Here's how the part is built. I have some questions about the finished solid (model axes, mm). Face numbers are marked on the shaded views. A direction names the side the tool comes from. Coordinates: 2 decimals unless noted, no trailing zeros. Write each loop counter-clockwise with the first axis right and the second up, starting at its lowest first coordinate (ties: lowest second). Pieces come first, ordered by that corner, then holes.
Item 1: For the marked faces 1 and 2, which set-ups out of +Z, -Z, +X, -X, +Y, -Y let a thin tool reach every point of the face, with its end or its side?
Item 2: If we section it at C-C (z = 23): Please give me the cut outline in (x, y).
Item 3: We'd pull the mould along Z, two halves only. Please class the marked faces 3, 4 and 5: +Z half, -Z half, draft (parallel to the pull), parting line (faces both ways), or undercut.
Item 4: If I drill on line 1 (Y direction, x = 12, z = -9); line 2 (Y direction, x = 22, z = 29); line 3 (Z direction, x = 0, y = -91.5), over which ranges is the centre line in solid material (lowest first)?
Item 5: If we section it at B-B (x = 0): Please give me the cut outline in (y, z), then the cut area to 3 significant figures.
Item 6: If we section it at D-D (y = -57.5): Please give me the cut outline in (x, z), then the cut area to 3 significant figures.
Item 7: I'm going to push flat-ended pins straight in: pin 1 Ø5 at (y, z) = (-63, -19.5) entering from -X; pin 2 Ø1.5 at (x, z) = (-12.5, 3.5) entering from -Y; pin 3 Ø10 at (x, z) = (35.96, -27.34) entering from +Y; pin 4 Ø6 at (x, y) = (24.5, -93.5) entering from -Z. Where does each tip first touch, or does it pass through?
Item 8: If we section it at A-A (z = 0): Please give me the cut outline in (x, y), then the cut area to 3 significant figures.
from build123d import *

# Parameters (mm, degrees)
F0_W     = 92.247778
F0_H     = 75.00481
F0_R     = 6.35
F1_DEPTH = 25.4
F2_R     = 31.75
F3_DEPTH = 76.2
F4_R     = 3.81
F5_DEPTH = 25.4


with BuildPart() as f1:
    # F0 (on Front) → F1 (new body)
    with BuildSketch(Plane.XZ):
        Rectangle(F0_W, F0_H)
        with Locations((-35.963889, -27.342405)):
            Circle(F0_R, mode=Mode.SUBTRACT)
        with Locations((35.963889, -27.342405)):
            Circle(F0_R, mode=Mode.SUBTRACT)
        with Locations((-35.963889, 27.342405)):
            Circle(F0_R, mode=Mode.SUBTRACT)
        with Locations((35.963889, 27.342405)):
            Circle(F0_R, mode=Mode.SUBTRACT)
    extrude(amount=F1_DEPTH)

    # F2 (on face) → F3 (join)
    with BuildSketch(Plane.XZ.offset(25.4)):
        Circle(F2_R)
    extrude(amount=F3_DEPTH)

    # F4 (on face) → F5 (join)
    with BuildSketch(Plane.XZ.offset(101.6)):
        Circle(F4_R)
    extrude(amount=F5_DEPTH)


solid = f1.part
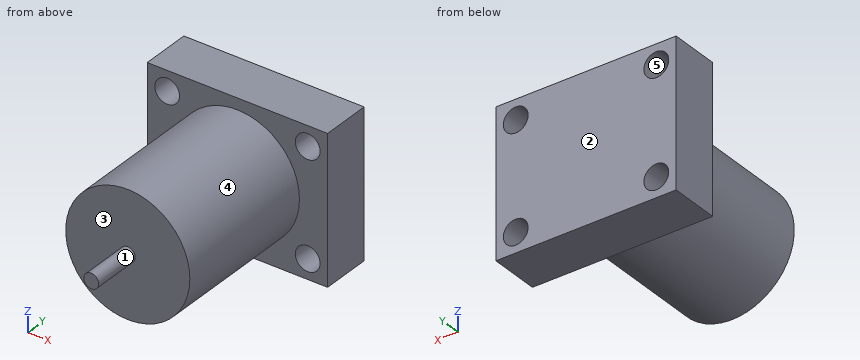
Answer list:
1. face 1: -Y
1. face 2: +Z, -Z, +X, -X, +Y
2. outline: (-46.12, -25.4) - (-40.6, -25.4) - (-40.6, 0) - (-46.12, 0) - close; (-31.33, -25.4) - (-21.89, -25.4) - (-21.89, -101.6) - (21.89, -101.6) - (21.89, -25.4) - (31.33, -25.4) - (31.33, 0) - (-31.33, 0) - close; (40.6, -25.4) - (46.12, -25.4) - (46.12, 0) - (40.6, 0) - close
3. face 3: draft
3. face 4: parting line
3. face 5: undercut
4. line 1: y = -101.6 to 0
4. line 2: y = -25.4 to 0
4. line 3: z = -31.75 to 31.75
5. outline: (-127, -3.81) - (-101.6, -3.81) - (-101.6, -31.75) - (-25.4, -31.75) - (-25.4, -37.5) - (0, -37.5) - (0, 37.5) - (-25.4, 37.5) - (-25.4, 31.75) - (-101.6, 31.75) - (-101.6, 3.81) - (-127, 3.81) - close
5. area: 6,940 mm2
6. outline: circle Ø63.5 at (0, 0)
6. area: 3,170 mm2
7. pin 1: stops at x = -26.82
7. pin 2: stops at y = -101.6
7. pin 3: passes through
7. pin 4: stops at z = -23.36
8. outline: (-46.12, -25.4) - (-31.75, -25.4) - (-31.75, -101.6) - (-3.81, -101.6) - (-3.81, -127) - (3.81, -127) - (3.81, -101.6) - (31.75, -101.6) - (31.75, -25.4) - (46.12, -25.4) - (46.12, 0) - (-46.12, 0) - close
8. area: 7,380 mm2
